from build123d import *

# Parameters (mm, degrees)
F0_W     = 10
F0_H     = 10
F0_W_2   = 4.63939
F0_H_2   = 4.217628
F1_DEPTH = 15


with BuildPart() as f1:
    # F0 (on Front) → F1 (new body, symmetric)
    with BuildSketch(Plane.XZ):
        with Locations((-12.142848, 20.394608)):
            Rectangle(F0_W, F0_H)
        with Locations((-12.185742, 20.606382)):
            Rectangle(F0_W_2, F0_H_2, mode=Mode.SUBTRACT)
    extrude(amount=F1_DEPTH, both=True)


solid = f1.part
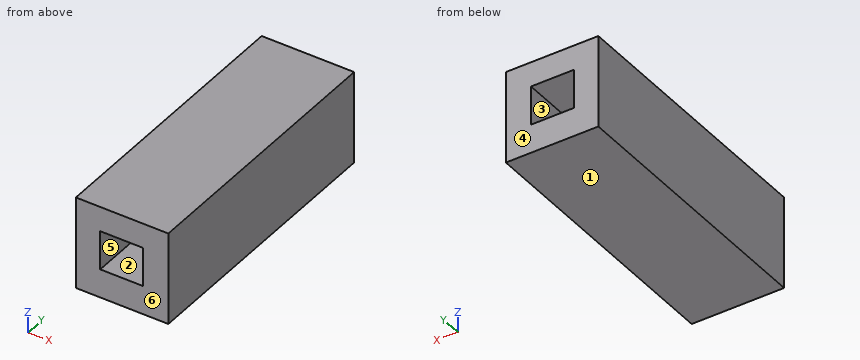
Check sheet for the modelled part. Datum: model origin and axes. Units: mm. Face numbers are marked on the shaded views. A direction names the side the tool comes from. Round coordinates to 2 decimals unless told otherwise and drop trailing zeros. Order: outer loops, then holes, each group sorted by start corner. A loop starts at its lowest first (then second) coordinate and runs counter-clockwise, first axis right, second up.
Q1. Set-up check for the marked faces 5 and 6: record each of +Z, -Z, +X, -X, +Y, -Y from which the full face is reachable in a straight line by a thin tool's end or side.
Filled sheet:
face 5: +Y, -Y
face 6: +Z, -Z, +X, -X, -Y
Q2. Cross-section at A-A, the plane x = -10.5. Enter the section's corners in (y, z).
Filled sheet:
outline: (-15, 15.39) - (15, 15.39) - (15, 18.5) - (-15, 18.5) - close; (-15, 22.72) - (15, 22.72) - (15, 25.39) - (-15, 25.39) - close
Q3. Cross-section at C-C, the plane z = 19. Enter the section's corners in (x, y), plus the area to 3 significant figures.
Filled sheet:
outline: (-17.14, -15) - (-14.51, -15) - (-14.51, 15) - (-17.14, 15) - close; (-9.87, -15) - (-7.14, -15) - (-7.14, 15) - (-9.87, 15) - close
area: 161 mm2
Q4. Cross-section at B-B, the plane y = -9.5. Enter the section's corners in (x, z), plus the area to 3 significant figures.
Filled sheet:
outline: (-17.14, 15.39) - (-7.14, 15.39) - (-7.14, 25.39) - (-17.14, 25.39) - close; hole (-14.51, 18.5) - (-9.87, 18.5) - (-9.87, 22.72) - (-14.51, 22.72) - close
area: 80.4 mm2
Q5. Scan lines: L1, parallel to X at y = -10.75, z = 19.5; L2, parallel to Z at x = -13.25, y = 11.25. Record each from-to range of solid material in increasing order.
Filled sheet:
L1: x = -17.14 to -14.51, -9.87 to -7.14
L2: z = 15.39 to 18.5, 22.72 to 25.39
Q6. Draft check along Z on the marked faces 1, 2, 3 and 4. Enter one of: pulls with the +Z half, pulls with the -Z half, needs draft (parallel to the pull), parting line crosses it, or undercut.
Filled sheet:
face 1: pulls with the -Z half
face 2: undercut
face 3: undercut
face 4: needs draft
